Can you work these out from the model? Positions are in its coordinate system, mm. Coordinates: 2 decimals unless noted, no trailing zeros. Order: outer loops, then holes, each group sorted by start corner. A loop starts at its lowest first (then second) coordinate and runs counter-clockwise, first axis right, second up.
```python
from build123d import *

# Parameters (mm, degrees)
SKETCH_W  = 304.8
SKETCH_H  = 304.8
SKETCH_R  = 14.318315
PAD_DEPTH = 10.000005


with BuildPart() as part:
    # Sketch → Pad (new body)
    with BuildSketch(Plane.XZ):
        Rectangle(SKETCH_W, SKETCH_H)
        with Locations((101.6, 101.6)):
            Circle(SKETCH_R, mode=Mode.SUBTRACT)
        with Locations((-101.6, 0)):
            Circle(SKETCH_R, mode=Mode.SUBTRACT)
        with Locations((101.6, 0)):
            Circle(SKETCH_R, mode=Mode.SUBTRACT)
        with Locations((0, 101.6)):
            Circle(SKETCH_R, mode=Mode.SUBTRACT)
        Circle(SKETCH_R, mode=Mode.SUBTRACT)
        with Locations((-101.6, 101.6)):
            Circle(SKETCH_R, mode=Mode.SUBTRACT)
        with BuildLine():
            ThreePointArc((-87.219092, -25.517974), (-125.319092, -63.617974), (-87.219092, -101.717974))
            Line((-87.219092, -101.717974), (90.580859, -101.717974))
            ThreePointArc((90.580859, -101.717974), (128.680859, -63.617974), (90.580859, -25.517974))
            Line((-87.219092, -25.517974), (90.580859, -25.517974))
        make_face(mode=Mode.SUBTRACT)
    extrude(amount=PAD_DEPTH)


solid = part.part
```
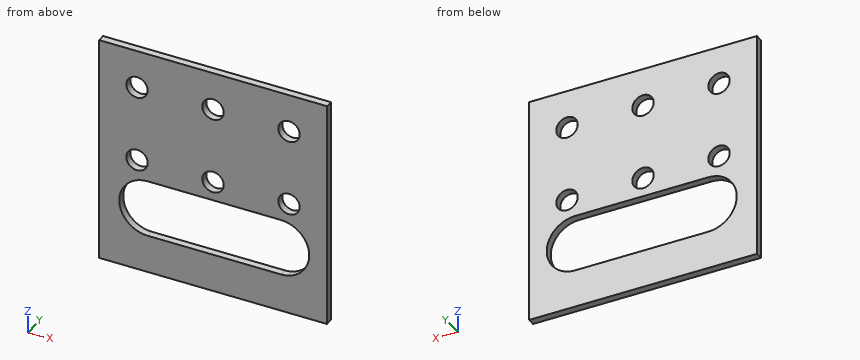
1. Imagine slicing it at A-A on x = 0. Please give me the cut outline in (y, z).
Completed:
outline: (-10, -152.4) - (0, -152.4) - (0, -101.72) - (-10, -101.72) - close; (-10, -25.52) - (0, -25.52) - (0, -14.32) - (-10, -14.32) - close; (-10, 14.32) - (0, 14.32) - (0, 87.28) - (-10, 87.28) - close; (-10, 115.92) - (0, 115.92) - (0, 152.4) - (-10, 152.4) - close
2. Please list where these lines run through material, in increasing order: probe 1 along Z at (x, y) = (0, -3.25); probe 2 along Z at (x, y) = (61, -1.5); probe 3 along Z at (x, y) = (-101.6, -4.5).
Completed:
probe 1: z = -152.4 to -101.72, -25.52 to -14.32, 14.32 to 87.28, 115.92 to 152.4
probe 2: z = -152.4 to -101.72, -25.52 to 152.4
probe 3: z = -152.4 to -98.9, -28.34 to -14.32, 14.32 to 87.28, 115.92 to 152.4
3. Imagine slicing it at D-D on z = -93. Please give me the cut outline in (x, y), then the cut area to 3 significant figures.
Completed:
outline: (-152.4, -10) - (-111.47, -10) - (-111.47, 0) - (-152.4, 0) - close; (114.84, -10) - (152.4, -10) - (152.4, 0) - (114.84, 0) - close
area: 785 mm2
4. I'm going to push a flat-ended pin straight in: pin 1 (23 mm diameter, centred on x = 101.6, z = 0, fed in from -Y). Where does the tip first touch, or does it pass through?
Completed:
pin 1: passes through
5. Imagine slicing it at C-C on y = -7.75. Please give me the cut outline in (x, z), then the cut area to 3 significant figures.
Completed:
outline: (-152.4, -152.4) - (152.4, -152.4) - (152.4, 152.4) - (-152.4, 152.4) - close; hole circle Ø28.64 at (-101.6, 0); hole circle Ø28.64 at (-101.6, 101.6); hole (-87.22, -101.72) - (90.58, -101.72) arc R38.1 ccw to (90.58, -25.52) - (-87.22, -25.52) arc R38.1 ccw to start; hole circle Ø28.64 at (0, 0); hole circle Ø28.64 at (0, 101.6); hole circle Ø28.64 at (101.6, 0); hole circle Ø28.64 at (101.6, 101.6)
area: 70,900 mm2
6. Imagine slicing it at B-B on z = 0. Please give me the cut outline in (x, y), then the cut area to 3 significant figures.
Completed:
outline: (-152.4, -10) - (-115.92, -10) - (-115.92, 0) - (-152.4, 0) - close; (-87.28, -10) - (-14.32, -10) - (-14.32, 0) - (-87.28, 0) - close; (14.32, -10) - (87.28, -10) - (87.28, 0) - (14.32, 0) - close; (115.92, -10) - (152.4, -10) - (152.4, 0) - (115.92, 0) - close
area: 2,190 mm2
